from build123d import *


with BuildPart() as part:
    # Skizze1 → Rotation1 (revolve)
    with BuildSketch(Plane.XY, mode=Mode.PRIVATE) as rotation1_sk:
        Polygon((0, 50), (0, 32.5), (5, 32.5), (5, 34.7), (8, 34.7), (8, 32.5), (20, 32.5), (20, 34.7), (23, 34.7), (23, 32.5), (30, 32.5), (30, 40), (200, 40), (200, 50), align=None)
    revolve(rotation1_sk.sketch.rotate(Axis((0, 0, 0), (1, 0, 0)), 90), axis=Axis((0, 0, 0), (1, 0, 0)))


solid = part.part
Design review of the part built by this model. Coordinates are the model's own, in mm. A direction names the side the tool comes from. Coordinates: 2 decimals unless noted, no trailing zeros. Order: outer loops, then holes, each group sorted by start corner. A loop starts at its lowest first (then second) coordinate and runs counter-clockwise, first axis right, second up. Notation, with made-up numbers: (42.5, 15) -> (70.5, 15) arc R16 cw to (70.5, 36) -> close; hole circle Ø8 at (79, -1). An arc over 180 degrees is marked (long way). One line per item, written item: value.
1) We need section D-D, the plane z = -37. Give the boundary of the cut face in (x, y), then the cut area to 3 significant figures.
Output values:
outline: (0, -33.63) -> (200, -33.63) -> (200, -15.2) -> (30, -15.2) -> (30, 15.2) -> (200, 15.2) -> (200, 33.63) -> (0, 33.63) -> close
area: 8,280 mm2
2) We need section C-C, the plane x = 117. Give the boundary of the cut face in (y, z), then the cut area to 3 significant figures.
Output values:
outline: circle Ø100 at (0, 0); hole circle Ø80 at (0, 0)
area: 2,830 mm2
3) To check wall thickness, follow probe 1 along X at (y, z) = (-17.5, 28); probe 2 along Y at (x, z) = (27, 0); probe 3 along Y at (x, z) = (22, 0). State the ranges of each line that lie inside material, in increasing order. Write a range as [from, to].
Output values:
probe 1: x = [0, 5], [8, 20], [23, 30]
probe 2: y = [-50, -32.5], [32.5, 50]
probe 3: y = [-50, -34.7], [34.7, 50]
4) We need section A-A, the plane z = 0. Give the boundary of the cut face in (x, y).
Output values:
outline: (0, -50) -> (200, -50) -> (200, -40) -> (30, -40) -> (30, -32.5) -> (23, -32.5) -> (23, -34.7) -> (20, -34.7) -> (20, -32.5) -> (8, -32.5) -> (8, -34.7) -> (5, -34.7) -> (5, -32.5) -> (0, -32.5) -> close; (0, 32.5) -> (5, 32.5) -> (5, 34.7) -> (8, 34.7) -> (8, 32.5) -> (20, 32.5) -> (20, 34.7) -> (23, 34.7) -> (23, 32.5) -> (30, 32.5) -> (30, 40) -> (200, 40) -> (200, 50) -> (0, 50) -> close
5) Machinability: for faces 1 (the face through (30, -33, 0)), 2 (the face through (8, -31, -10.4)), 3 (the face through (26.55, -9.76, 31)), which of the approach directions +Z, -Z, +X, -X, +Y, -Y give a long, thin tool a straight path to every point of the face, cutting with its end or side? Answer none if there is none.
Output values:
face 1: +X
face 2: none
face 3: +X, -X
6) Clearance check with flat-ended pins moving along their axes: P1, Ø2, axis at x = 107.5, y = -35.5, coming from the -Z side; P2, Ø1.5, axis at x = 176, z = -5.5, coming from the +Y side; P3, Ø1, axis at x = 148, y = 27.5, coming from the -Z side; P4, Ø8, axis at y = -10.5, z = -28.5, coming from the -X side. State where each tip first meets the part, or that it passes through.
Output values:
P1: stops at z = -36.19
P2: stops at y = 49.77
P3: stops at z = -42.08
P4: stops at x = 0
7) Draft analysis for pull direction X (two halves, no side actions). For faces 4 (the face through (6.521, -34.405, -4.517)), 5 (the face through (116.19, -1.76, -39.96)), 6 (the face through (200, -34, 22)), state which applies: +X half, -X half, draft (parallel to the pull), parting line (faces both ways), or undercut.
Output values:
face 4: undercut
face 5: draft
face 6: +X half
